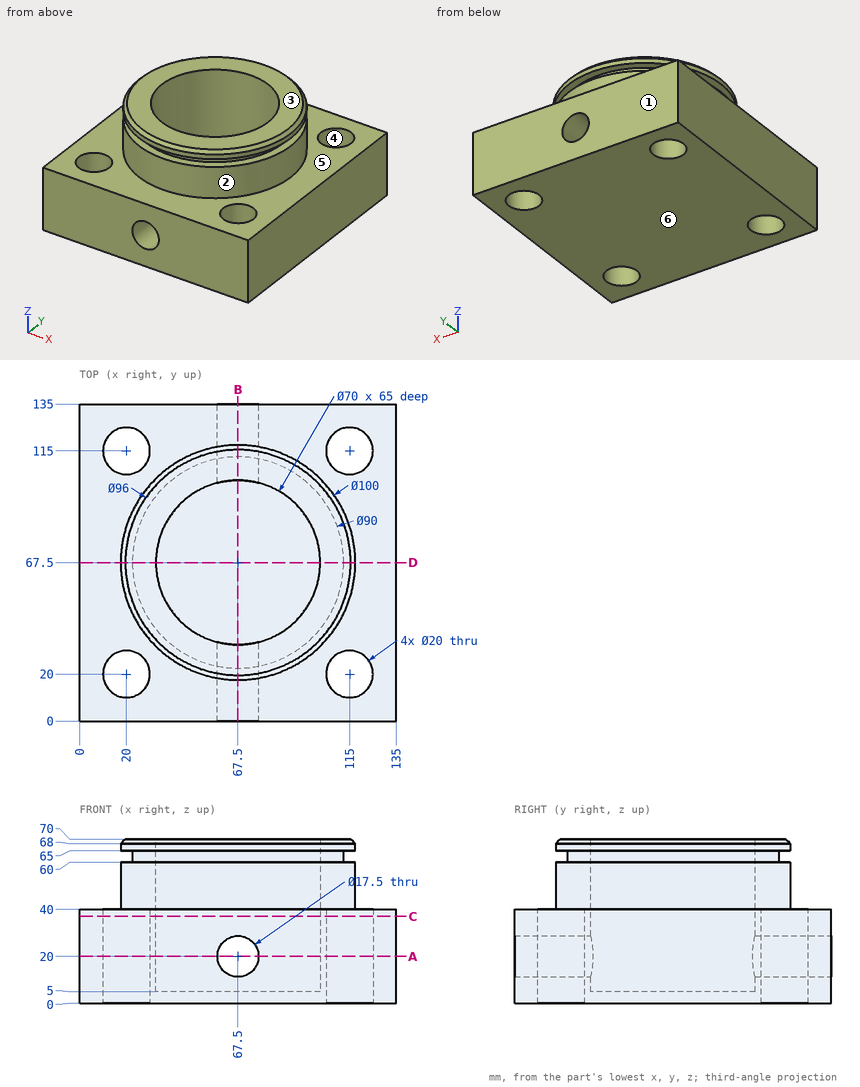
The figure shows three views and two pictorial views of one solid part (mm, origin at its lowest corner). Answer the questions. A direction names the side the tool comes from. Round coordinates to 2 decimals unless told otherwise and drop trailing zeros. Order: outer loops, then holes, each group sorted by start corner. A loop starts at its lowest first (then second) coordinate and runs counter-clockwise, first axis right, second up.
Q1. A tool of negligible diameter and unlimited length cuts with its end or side. For the marked faces 5 and 6, from which of +Z, -Z, +X, -X, +Y, -Y can it reach the whole face along a straight path? Write none if from no direction.
Solution:
face 5: +Z
face 6: -Z, +X, -X, +Y, -Y
Q2. A cutting plane is placed at D-D, the plane y = 67.5. Determine the outline of the cut face in (x, z).
Solution:
outline: (0, 0) - (135, 0) - (135, 40) - (117.5, 40) - (117.5, 60) - (112.5, 60) - (112.5, 65) - (117.5, 65) - (117.5, 68) - (115.5, 70) - (102.5, 70) - (102.5, 5) - (32.5, 5) - (32.5, 70) - (19.5, 70) - (17.5, 68) - (17.5, 65) - (22.5, 65) - (22.5, 60) - (17.5, 60) - (17.5, 40) - (0, 40) - close
Q3. Find the intervals of material crossed by line 1 along Y through (x, z) = (20, 11.5); line 2 along Y through (x, z) = (67.5, 33); line 3 along Y through (x, z) = (67.5, 44), in increasing order.
Solution:
line 1: y = 0 to 10, 30 to 105, 125 to 135
line 2: y = 0 to 32.5, 102.5 to 135
line 3: y = 17.5 to 32.5, 102.5 to 117.5
Q4. A cutting plane is placed at B-B, the plane x = 67.5. Count the separate pieces of the cut face and the enclosed holes in it, then the cut area to 3 significant figures.
Solution:
separate pieces: 3
enclosed holes: 0
area: 2,660 mm2
Q5. Given pin 1 Ø10 at (x, z) = (68.5, 60.5) entering from -Y; pin 2 Ø8 at (y, z) = (20, 54.5) entering from +X; pin 3 Ø3 at (x, y) = (96.5, 14.5) entering from +Z, each flat-ended and moving along its own axis, determine where each tip first touches the part or whether it passes through.
Solution:
pin 1: stops at y = 17.5
pin 2: stops at x = 92.15
pin 3: stops at z = 40
Q6. A cutting plane is placed at C-C, the plane z = 37. Determine the outline of the cut face in (x, y), then the cut area to 3 significant figures.
Solution:
outline: (0, 0) - (135, 0) - (135, 135) - (0, 135) - close; hole circle Ø20 at (20, 20); hole circle Ø20 at (20, 115); hole circle Ø70 at (67.5, 67.5); hole circle Ø20 at (115, 20); hole circle Ø20 at (115, 115)
area: 13,100 mm2
Q7. A cutting plane is placed at A-A, the plane z = 20. Determine the outline of the cut face in (x, y), then the cut area to 3 significant figures.
Solution:
outline: (0, 0) - (58.75, 0) - (58.75, 33.61) arc R35 cw to (58.75, 101.39) - (58.75, 135) - (0, 135) - close; (76.25, 0) - (135, 0) - (135, 135) - (76.25, 135) - (76.25, 101.39) arc R35 cw to (76.25, 33.61) - close; hole circle Ø20 at (20, 20); hole circle Ø20 at (20, 115); hole circle Ø20 at (115, 20); hole circle Ø20 at (115, 115)
area: 12,000 mm2
Q8. The mould has two halves that part along Y. Classify the marked faces 1, 2, 3 and 4: pulls with the +Y half, pulls with the -Y half, needs draft (parallel to the pull), parting line crosses it, or undercut.
Solution:
face 1: pulls with the +Y half
face 2: parting line crosses it
face 3: needs draft
face 4: undercut
